For this review, take the finished solid that the model builds, in its own axes (mm). A direction names the side the tool comes from. Coordinates: 2 decimals unless noted, no trailing zeros. Order: outer loops, then holes, each group sorted by start corner. A loop starts at its lowest first (then second) coordinate and runs counter-clockwise, first axis right, second up. Notation, with made-up numbers: (37.5, -35.75) -> (62.5, -35.75) arc R31 ccw to (62.5, -7.75) -> close; hole circle Ø9 at (47, -37). An arc over 180 degrees is marked (long way). Return JSON: item names as keys, results as strings. Group by question number.
Item 1: For line 1 along Y through (x, z) = (-16, 60.5); line 2 along Z through (x, y) = (12, -361); line 3 along X through (y, z) = (-387, 67.5), list the stretches that pass through material, from the lowest coordinate up.
Item 2: Machinability: for faces 4 (the flat face through (-9, -405, 45)), 5 (the flat face through (-8, -1.6, 45)), which of the approach directions +Z, -Z, +X, -X, +Y, -Y give a long, thin tool a straight path to every point of the face, cutting with its end or side? Answer none if there is none.
Item 3: Take a section at A-A (z = 55.5). Write out the cut boundary in (x, y), then the cut area to 3 significant figures.
Item 4: Take a section at B-B (x = -47). Write out the cut boundary in (y, z), then the cut area to 3 significant figures.
Item 5: Draft analysis for pull direction Y (two halves, no side actions). For faces 1 (the flat face through (-30.63, -199.665, 36.504)), 2 (the flat face through (13, -205, 1.6)), 3 (the flat face through (-9, 0, 45)), state which applies: +Y half, -Y half, draft (parallel to the pull), parting line (faces both ways), or undercut.
Item 6: Insertion check: pin 1 (0.5 mm diameter, centred on y = -404.5, z = 37.5, fed in from +X); pin 2 (4 mm diameter, centred on x = -5, y = -241, fed in from +Z); pin 3 (6 mm diameter, centred on y = -327, z = 54, fed in from +X). Each pin has a flat end and moves straight along its axis. Give the tip position at first contact, or say it passes through.
Item 7: Take a section at C-C (y = -240). Write out the cut boundary in (x, z).
```python
from build123d import *

# Parameters (mm, degrees)
F1_DEPTH = 405
F4_DEPTH = 401.8


with BuildPart() as f1:
    # F0 (on Front) → F1 (new body)
    with BuildSketch(Plane.XZ):
        Polygon((-60.4151734448, 72), (0, 0), (25, 0), (25, 30), (10, 30), (10, 43), (25, 43), (25, 72), align=None)
    extrude(amount=F1_DEPTH)

    # F3 (on offset) → F4 (cut)
    with BuildSketch(Plane.XZ.offset(403.4)):
        Polygon((29.3578643668, 73.0284601755), (-59.1895023358, 73.0284601755), (0.746092253, 1.6), (25, 1.6), align=None)
    extrude(amount=-F4_DEPTH, mode=Mode.SUBTRACT)


solid = f1.part
```
Findings below:
{
 "1": {"line 1": "y = -405 to -403.4, -1.6 to 0", "line 2": "z = 0 to 1.6", "line 3": "x = -56.64 to -54.55"},
 "2": {"face 4": "+Z, -Z, +X, -X, -Y", "face 5": "+Z, +X"},
 "3": {"outline": "(-46.57, -405) -> (25, -405) -> (25, -403.4) -> (-44.48, -403.4) -> (-44.48, -1.6) -> (25, -1.6) -> (25, 0) -> (-46.57, 0) -> close", "area": "1,070 mm2"},
 "4": {"outline": "(-405, 56.01) -> (0, 56.01) -> (0, 72) -> (-1.6, 72) -> (-1.6, 58.5) -> (-403.4, 58.5) -> (-403.4, 72) -> (-405, 72) -> close", "area": "1,050 mm2"},
 "5": {"face 1": "draft", "face 2": "undercut", "face 3": "+Y half"},
 "6": {"pin 1": "stops at x = 10", "pin 2": "stops at z = 10.83", "pin 3": "stops at x = -40.71"},
 "7": {"outline": "(-60.42, 72) -> (0, 0) -> (25, 0) -> (25, 1.6) -> (0.75, 1.6) -> (-58.33, 72) -> close"}
}
